```python
from build123d import *

# Parameters (mm, degrees)
F0_R     = 11.034718
F1_DEPTH = 63.5


with BuildPart() as f1:
    # F0 (on Top) → F1 (new body)
    with BuildSketch(Plane.XY):
        with BuildLine():
            Line((-32.078517, 45.276365), (-28.134993, 34.4225))
            ThreePointArc((-28.134993, 34.4225), (-30.590232, 32.037975), (-32.865392, 29.481061))
            Line((-32.865392, 29.481061), (-43.88094, 32.947393))
            Line((-43.88094, 32.947393), (-46.882508, 28.235875))
            Line((-46.882508, 28.235875), (-39.085573, 19.717333))
            ThreePointArc((-39.085573, 19.717333), (-40.441399, 16.57474), (-41.564885, 13.341794))
            Line((-41.564885, 13.341794), (-53.068432, 12.328799))
            Line((-53.068432, 12.328799), (-54.038499, 6.827273))
            Line((-54.038499, 6.827273), (-43.575165, 1.940925))
            ThreePointArc((-43.575165, 1.940925), (-43.625167, -1.481305), (-43.425937, -4.898097))
            Line((-43.425937, -4.898097), (-53.666173, -10.236199))
            Line((-53.666173, -10.236199), (-52.457055, -15.690175))
            Line((-52.457055, -15.690175), (-40.920271, -16.200428))
            ThreePointArc((-40.920271, -16.200428), (-39.656836, -19.381291), (-38.165222, -22.461753))
            Line((-38.165222, -22.461753), (-45.583163, -31.312284))
            Line((-45.583163, -31.312284), (-42.378938, -35.888392))
            Line((-42.378938, -35.888392), (-31.525073, -31.944868))
            ThreePointArc((-31.525073, -31.944868), (-29.140548, -34.400106), (-26.583635, -36.675266))
            Line((-26.583635, -36.675266), (-30.049966, -47.690814))
            Line((-30.049966, -47.690814), (-25.338448, -50.692383))
            Line((-25.338448, -50.692383), (-16.819906, -42.895447))
            ThreePointArc((-16.819906, -42.895447), (-13.677313, -44.251274), (-10.444367, -45.374759))
            Line((-10.444367, -45.374759), (-9.431372, -56.878306))
            Line((-9.431372, -56.878306), (-3.929846, -57.848374))
            Line((-3.929846, -57.848374), (0.956502, -47.38504))
            ThreePointArc((0.956502, -47.38504), (4.378732, -47.435041), (7.795524, -47.235812))
            Line((7.795524, -47.235812), (13.133626, -57.476047))
            Line((13.133626, -57.476047), (18.587602, -56.26693))
            Line((18.587602, -56.26693), (19.097855, -44.730146))
            ThreePointArc((19.097855, -44.730146), (22.278718, -43.46671), (25.35918, -41.975097))
            Line((25.35918, -41.975097), (34.209711, -49.393037))
            Line((34.209711, -49.393037), (38.785819, -46.188812))
            Line((38.785819, -46.188812), (34.842295, -35.334948))
            ThreePointArc((34.842295, -35.334948), (37.297533, -32.950422), (39.572693, -30.393509))
            Line((39.572693, -30.393509), (50.588241, -33.859841))
            Line((50.588241, -33.859841), (53.589809, -29.148323))
            Line((53.589809, -29.148323), (45.792874, -20.629781))
            ThreePointArc((45.792874, -20.629781), (47.1487, -17.487187), (48.272186, -14.254241))
            Line((48.272186, -14.254241), (59.775733, -13.241247))
            Line((59.775733, -13.241247), (60.7458, -7.739721))
            Line((60.7458, -7.739721), (50.282467, -2.853372))
            ThreePointArc((50.282467, -2.853372), (50.332468, 0.568858), (50.133239, 3.985649))
            Line((50.133239, 3.985649), (60.373474, 9.323751))
            Line((60.373474, 9.323751), (59.164357, 14.777727))
            Line((59.164357, 14.777727), (47.627572, 15.28798))
            ThreePointArc((47.627572, 15.28798), (46.364137, 18.468843), (44.872523, 21.549305))
            Line((44.872523, 21.549305), (52.290464, 30.399837))
            Line((52.290464, 30.399837), (49.086239, 34.975944))
            Line((49.086239, 34.975944), (38.232375, 31.03242))
            ThreePointArc((38.232375, 31.03242), (35.847849, 33.487659), (33.290936, 35.762819))
            Line((33.290936, 35.762819), (36.757268, 46.778367))
            Line((36.757268, 46.778367), (32.045749, 49.779935))
            Line((32.045749, 49.779935), (23.527208, 41.983))
            ThreePointArc((23.527208, 41.983), (20.384614, 43.338826), (17.151668, 44.462311))
            Line((17.151668, 44.462311), (16.138674, 55.965858))
            Line((16.138674, 55.965858), (10.637148, 56.935926))
            Line((10.637148, 56.935926), (5.750799, 46.472592))
            ThreePointArc((5.750799, 46.472592), (2.328569, 46.522594), (-1.088223, 46.323364))
            Line((-1.088223, 46.323364), (-6.426325, 56.5636))
            Line((-6.426325, 56.5636), (-11.8803, 55.354482))
            Line((-11.8803, 55.354482), (-12.390553, 43.817698))
            ThreePointArc((-12.390553, 43.817698), (-15.571416, 42.554263), (-18.651878, 41.062649))
            Line((-18.651878, 41.062649), (-27.50241, 48.48059))
            Line((-27.50241, 48.48059), (-32.078517, 45.276365))
        make_face()
        with Locations((3.353651, -0.456224)):
            Circle(F0_R, mode=Mode.SUBTRACT)
    extrude(amount=F1_DEPTH)


solid = f1.part
```
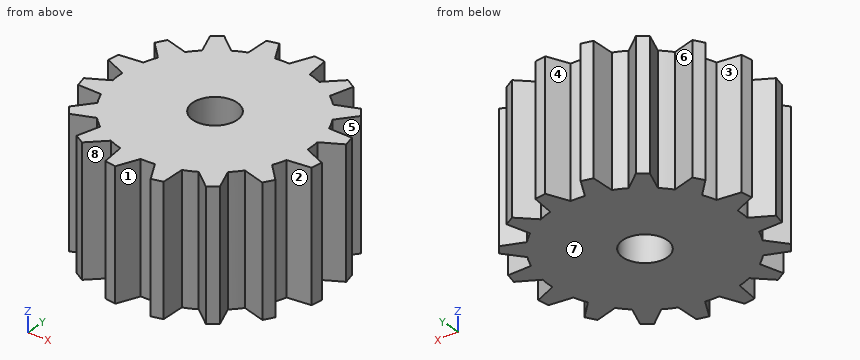
Can you work these out from the model? Positions are in its coordinate system, mm. Face numbers are marked on the shaded views. A direction names the side the tool comes from. Round coordinates to 2 decimals unless told otherwise and drop trailing zeros. Loops run counter-clockwise (first coordinate to the right, second up) from the corner with the lowest first, then second, coordinate; pieces in that order, holes last. Notation, with made-up numbers: (83, -19.5) -> (101, -19.5) arc R10 cw to (101, -10.5) -> close; hole circle Ø10 at (-25, -6.75). An arc over 180 degrees is marked (long way). One line per item, written item: value. Start each with the question number.
1. If I drill on probe 1 along Y at (x, z) = (46, 29); probe 2 along Y at (x, z) = (48.5, 25); probe 3 along X at (y, z) = (8.5, 25), over which ranges is the centre line in solid material (lowest first)?
2. If we mould it in two halves opening along Y, with no side actions, what happens to the marked faces 5, 6, 7 and 8? For each: pulls with the +Y half, pulls with the -Y half, needs draft (parallel to the pull), parting line crosses it, or undercut.
3. For the marked faces 1, 2, 3 and 4, which set-ups out of +Z, -Z, +X, -X, +Y, -Y let a thin tool reach every point of the face, with its end or its side?
4. If we section it at B-B, the plane y = 26.5: Write out the boundary of the cut face in (x, z), then the cut area to 3 significant figures.
5. For pin 1 (4 mm diameter, centred on x = -35, z = 33, fed in from +Y); pin 2 (10 mm diameter, centred on x = -5.5, y = 28.5, fed in from -Z); pin 3 (3 mm diameter, centred on y = 14, z = 11, fed in from +X); pin 4 (2 mm diameter, centred on y = -30.5, z = 20.5, fed in from +X), each with a flat end and sliding along its axis, tell me the tip position at first contact or that it passes through.
6. If we section it at A-A, the plane y = -39: Write out the boundary of the cut face in (x, z).
Calculated:
1. probe 1: y = -32.42 to -20.86, -20.19 to 19.28, 22.89 to 33.85
1. probe 2: y = -33.2 to -23.59, -14.23 to 15.25, 25.88 to 34.76
1. probe 3: x = -53.74 to -3.09, 9.8 to 58.79
2. face 5: undercut
2. face 6: pulls with the +Y half
2. face 7: needs draft
2. face 8: pulls with the -Y half
3. face 1: +Z, -Z, -Y
3. face 2: +Z, -Z, +X
3. face 3: +Z, -Z, -X
3. face 4: +Z, -Z, +Y
4. outline: (-45.29, 0) -> (49.02, 0) -> (49.02, 63.5) -> (-45.29, 63.5) -> close
4. area: 5,990 mm²
5. pin 1: stops at y = 30.78
5. pin 2: stops at z = 0
5. pin 3: stops at x = 59.67
5. pin 4: stops at x = 53.37
6. outline: (-27.32, 0) -> (36.17, 0) -> (36.17, 63.5) -> (-27.32, 63.5) -> close
